Read the model definition and answer for the solid it produces. Units are mm, in the model's axes. Face numbers are marked on the shaded views. A direction names the side the tool comes from. Round coordinates to 2 decimals unless told otherwise and drop trailing zeros. Order: outer loops, then holes, each group sorted by start corner. A loop starts at its lowest first (then second) coordinate and runs counter-clockwise, first axis right, second up.
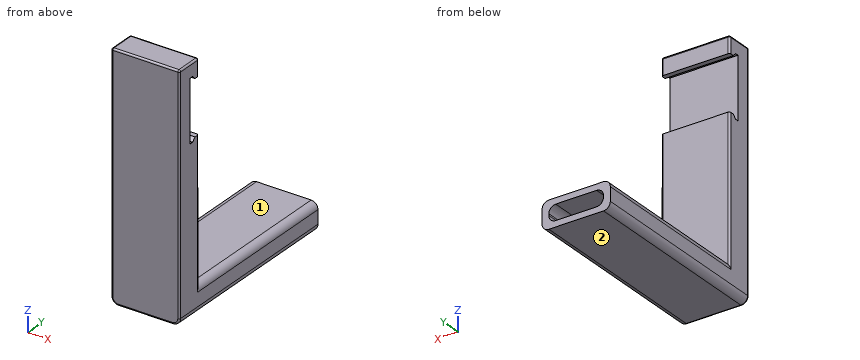
from build123d import *

# Parameters (mm, degrees)
SKETCH1_W           = 20
SKETCH1_H           = 8
BOSS_EXTRUDE2_DEPTH = 70
SKETCH3_W           = 20
SKETCH3_H           = 8
BOSS_EXTRUDE3_DEPTH = 50
SKETCH4_W           = 16
SKETCH4_H           = 4.5
CUT_EXTRUDE2_DEPTH  = 40
FILLET1_R           = 2
CUT_EXTRUDE3_DEPTH  = 28
FILLET3_R           = 0.5
FILLET4_R           = 2


with BuildPart() as part:
    # Sketch1 → Boss-Extrude2 (new body)
    with BuildSketch(Plane.XY):
        Rectangle(SKETCH1_W, SKETCH1_H)
    extrude(amount=BOSS_EXTRUDE2_DEPTH)

    # Sketch3 → Boss-Extrude3 (add)
    with BuildSketch(Plane(origin=(0, 4, 0), x_dir=(1, 0, 0), z_dir=(0, 1, 0))):
        with Locations((0, -4)):
            Rectangle(SKETCH3_W, SKETCH3_H)
    extrude(amount=BOSS_EXTRUDE3_DEPTH)

    # Sketch4 → Cut-Extrude2 (cut)
    with BuildSketch(Plane(origin=(0, 54, 0), x_dir=(1, 0, 0), z_dir=(0, 1, 0))):
        with Locations((0, -4)):
            Rectangle(SKETCH4_W, SKETCH4_H)
    extrude(amount=-CUT_EXTRUDE2_DEPTH, mode=Mode.SUBTRACT)

    # Fillet1
    fillet1_edges = [part.edges().sort_by_distance(p)[0] for p in [
        (-10, 29, 8),
        (10, 29, 8),
        (-10, 25, 0),
        (10, 25, 0),
    ]]
    fillet(fillet1_edges, radius=FILLET1_R)

    # Sketch5 → Cut-Extrude3 (cut)
    with BuildSketch(Plane.ZY.offset(10)):
        Polygon((65, 4), (65, 2.5), (66, 1.5), (66, 0.5), (48, 0.5), (48, 1.5), (49, 2.5), (49, 4), align=None)
    extrude(amount=-CUT_EXTRUDE3_DEPTH, mode=Mode.SUBTRACT)

    # Fillet3
    fillet3_edges = [part.edges().sort_by_distance(p)[0] for p in [
        (-10, 0, 70),
        (0, -4, 70),
        (0, -4, 0),
        (-9.414213562, -4, 0.585786438),
        (10, 0, 70),
        (9.414213562, -4, 0.585786438),
        (10, -4, 36),
        (-10, 4, 27.5),
        (-10, -4, 36),
        (-10, 4, 67.5),
        (10, 4, 67.5),
        (10, 4, 27.5),
        (0, 4, 70),
    ]]
    fillet(fillet3_edges, radius=FILLET3_R)

    # Fillet4
    fillet4_edges = [part.edges().sort_by_distance(p)[0] for p in [
        (8, 34, 1.75),
        (8, 34, 6.25),
        (-8, 34, 6.25),
        (-8, 34, 1.75),
    ]]
    fillet(fillet4_edges, radius=FILLET4_R)


solid = part.part
Q1. A cutting plane is placed at A-A, the plane y = 49. Give the vertices of the cut face in (x, z).
Outcome:
outline: (-10, 2) arc R2 ccw to (-8, 0) - (8, 0) arc R2 ccw to (10, 2) - (10, 6) arc R2 ccw to (8, 8) - (-8, 8) arc R2 ccw to (-10, 6) - close; hole (-8, 3.75) arc R2 ccw to (-6, 1.75) - (6, 1.75) arc R2 ccw to (8, 3.75) - (8, 4.25) arc R2 ccw to (6, 6.25) - (-6, 6.25) arc R2 ccw to (-8, 4.25) - close
Q2. For the marked faces 1 and 2, determine the directions among +Z, -Z, +X, -X, +Y, -Y from which every point of the face is accessible in a straight line to the end or side of a thin tool.
Outcome:
face 1: +Z, +X, -X, +Y
face 2: -Z, +X, -X, +Y, -Y
Q3. A cutting plane is placed at C-C, the plane y = 10.5. Give the vertices of the cut face in (x, z), plus the area to 3 significant figures.
Outcome:
outline: (-10, 2) arc R2 ccw to (-8, 0) - (8, 0) arc R2 ccw to (10, 2) - (10, 6) arc R2 ccw to (8, 8) - (-8, 8) arc R2 ccw to (-10, 6) - close
area: 157 mm2
Q4. Flat-ended cylindrical pins translate along their axes: pin 1 (5 mm diameter, centred on x = 1, z = 67.5, fed in from +Y); pin 2 (2 mm diameter, centred on x = 0.5, y = 35, fed in from +Z); pin 3 (6 mm diameter, centred on y = 8.5, z = 63, fed in from -X); pin 4 (4 mm diameter, centred on y = 27.5, z = 8, fed in from +X). Find the tip coordinate at first contact, or state that the pin passes through.
Outcome:
pin 1: stops at y = 4
pin 2: stops at z = 8
pin 3: passes through
pin 4: stops at x = 10
Q5. A cutting plane is placed at B-B, the plane z = 32.5. Give the vertices of the cut face in (x, y), plus the area to 3 significant figures.
Outcome:
outline: (-10, -3.5) arc R0.5 ccw to (-9.5, -4) - (9.5, -4) arc R0.5 ccw to (10, -3.5) - (10, 3.5) arc R0.5 ccw to (9.5, 4) - (-9.5, 4) arc R0.5 ccw to (-10, 3.5) - close
area: 160 mm2
Q6. A cutting plane is placed at D-D, the plane x = -2. Give the vertices of the cut face in (y, z).
Outcome:
outline: (-4, 0.5) arc R0.5 ccw to (-3.5, 0) - (54, 0) - (54, 1.75) - (14, 1.75) - (14, 6.25) - (54, 6.25) - (54, 8) - (4, 8) - (4, 49) - (2.5, 49) - (1.5, 48) - (0.5, 48) - (0.5, 66) - (1.5, 66) - (2.5, 65) - (4, 65) - (4, 69.5) arc R0.5 ccw to (3.5, 70) - (-3.5, 70) arc R0.5 ccw to (-4, 69.5) - close
Q7. Straight lines are drawn through the part: probe 1 along Z at (x, y) = (-0.75, 3.5); probe 2 along Z at (x, y) = (3.5, 27); probe 3 along Y at (x, z) = (-7, 47). For each, find the intervals that lie inside material, in ascending order.
Outcome:
probe 1: z = 0 to 49, 65 to 70
probe 2: z = 0 to 1.75, 6.25 to 8
probe 3: y = -4 to 4
